Verification items for this drawing (mm, ordinates from the low corner). A direction names the side the tool comes from. Coordinates: 2 decimals unless noted, no trailing zeros. Order: outer loops, then holes, each group sorted by start corner. A loop starts at its lowest first (then second) coordinate and runs counter-clockwise, first axis right, second up. Notation, with made-up numbers: (88, -8) -> (105, -8) arc R21 ccw to (105, -3) -> close; hole circle Ø2 at (8, -17). An arc over 180 degrees is marked (long way). Write item = value, one per line. Start each with the question number.
1. Cross-section at B-B on y = 19.05. Record the cut outline in (x, z) (1 decimal), plus the area to 3 significant figures.
2. Release check for a two-part mould opening along X. For the marked faces 3, 4 and 5 record: +X half, -X half, draft (parallel to the pull), parting line (faces both ways), or undercut.
3. Set-up check for the marked faces 1 and 2: record each of +Z, -Z, +X, -X, +Y, -Y from which the full face is reachable in a straight line by a thin tool's end or side.
4. Thickness scan on line 1 along Y through (x, z) = (19, 34) (1 decimal); line 2 along Y through (x, z) = (19, 20) (1 decimal). Record the ranges inside material, lowest first. Write a range as from..to.
5. Cross-section at C-C on x = 5.5. Record the cut outline in (y, z) (1 decimal), plus the area to 3 significant figures.
6. Cross-section at A-A on x = 19.05. Record the cut outline in (y, z) (1 decimal).
7. Go/stop test with flat-tipped pins: P1, Ø8, axis at x = 19.05, y = 4.76, coming from the -Z side (1 decimal); P2, Ø3, axis at x = 6.68, y = 26.19, coming from the -Z side; P3, Ø1, axis at y = 10.5, z = 4.5, coming from the -X side; P4, Ø8, axis at y = 9.5, z = 27, coming from the -X side. Record where each tip stops, or that it passes through.
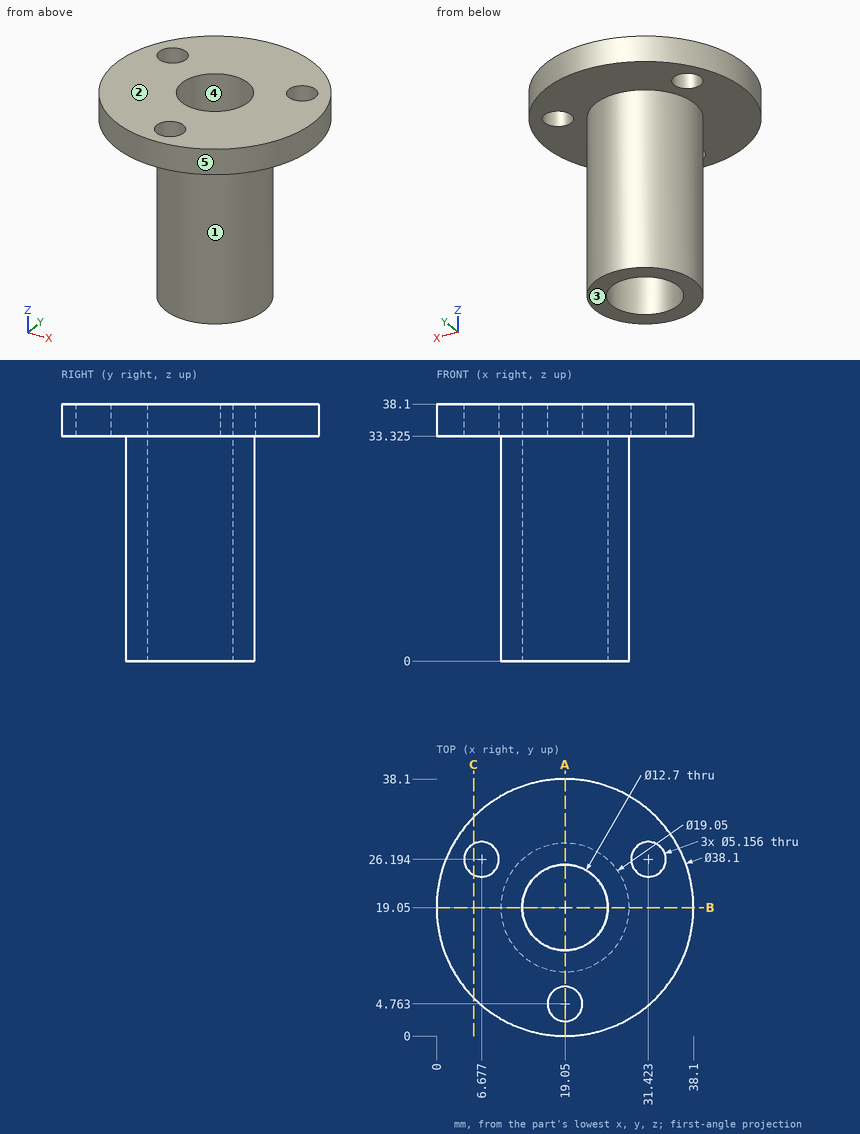
Worked out:
q1.outline = (0, 33.3) -> (9.5, 33.3) -> (9.5, 0) -> (12.7, 0) -> (12.7, 38.1) -> (0, 38.1) -> close; (25.4, 0) -> (28.6, 0) -> (28.6, 33.3) -> (38.1, 33.3) -> (38.1, 38.1) -> (25.4, 38.1) -> close
q1.area = 333 mm²
q2.face_3 = draft
q2.face_4 = undercut
q2.face_5 = parting line
q3.face_1 = -Z
q3.face_2 = +Z, +X, -X, +Y, -Y
q4.line_1 = 0..2.2, 7.3..12.7, 25.4..38.1
q4.line_2 = 9.5..12.7, 25.4..28.6
q5.outline = (5.7, 33.3) -> (23.9, 33.3) -> (23.9, 38.1) -> (5.7, 38.1) -> close; (28.5, 33.3) -> (32.4, 33.3) -> (32.4, 38.1) -> (28.5, 38.1) -> close
q5.area = 106 mm²
q6.outline = (0, 33.3) -> (2.2, 33.3) -> (2.2, 38.1) -> (0, 38.1) -> close; (7.3, 33.3) -> (9.5, 33.3) -> (9.5, 0) -> (12.7, 0) -> (12.7, 38.1) -> (7.3, 38.1) -> close; (25.4, 0) -> (28.6, 0) -> (28.6, 33.3) -> (38.1, 33.3) -> (38.1, 38.1) -> (25.4, 38.1) -> close
q7.P1 = 33.3
q7.P2 = through
q7.P3 = 13.96
q7.P4 = 11.31
